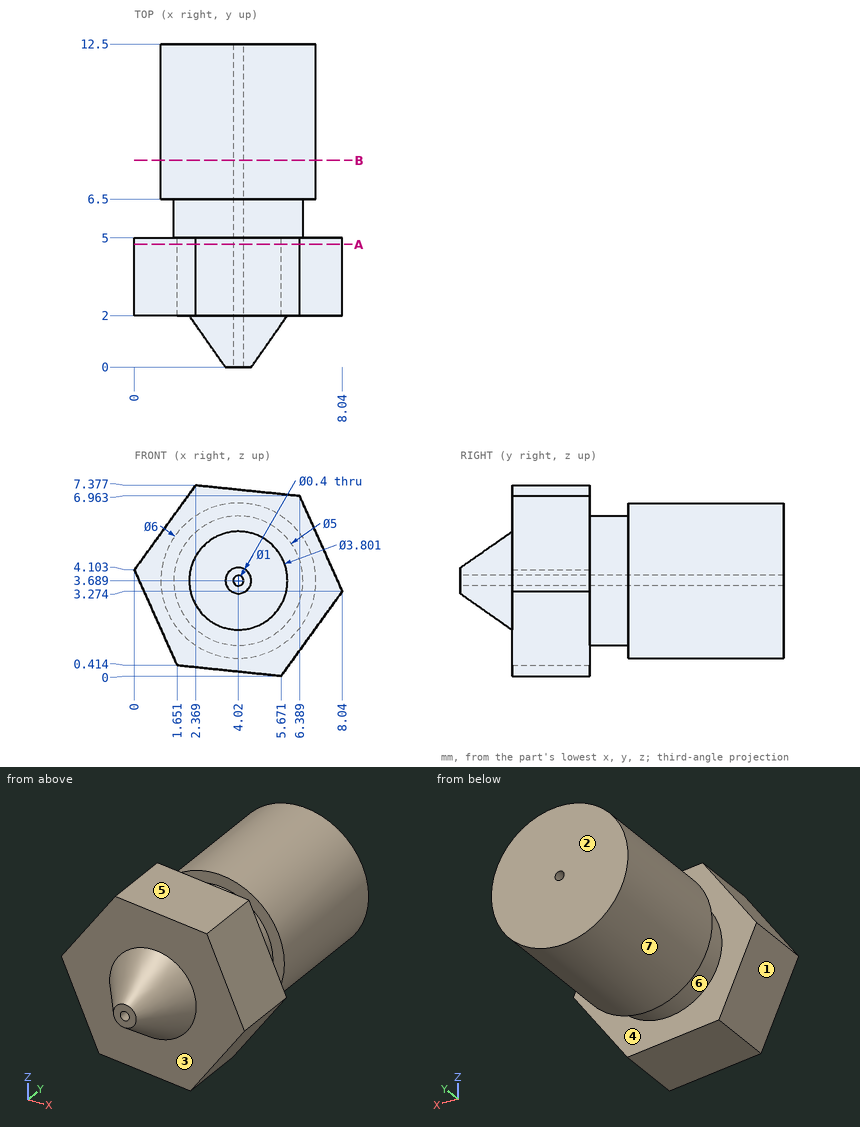
The drawing under review shows one solid part. Ordinate dimensions are in mm from its lowest x, y, z. A direction names the side the tool comes from. Round coordinates to 2 decimals unless told otherwise and drop trailing zeros. Order: outer loops, then holes, each group sorted by start corner. A loop starts at its lowest first (then second) coordinate and runs counter-clockwise, first axis right, second up. Notation, with made-up numbers: (-34.75, 36.5) -> (4.25, 36.5) arc R26 cw to (4.25, 67.5) -> close; hole circle Ø8 at (-14.75, 12.25). An arc over 180 degrees is marked (long way). Use a Markdown table: item, result.
Item 1: Draft analysis for pull direction Y (two halves, no side actions). For the marked faces 1, 2, 3 and 4, state which applies: +Y half, -Y half, draft (parallel to the pull), parting line (faces both ways), or undercut.
Resolved:
| item | result |
|---|---|
| face 1 | draft |
| face 2 | +Y half |
| face 3 | -Y half |
| face 4 | undercut |
Item 2: For pin 1 (1.5 mm diameter, centred on x = 2.5, z = 4, fed in from -Y); pin 2 (1 mm diameter, centred on y = 10, z = 5.5, fed in from -X); pin 3 (2 mm diameter, centred on x = 3.5, z = 2.5, fed in from -Y); pin 4 (2 mm diameter, centred on y = 9, z = 2.5, fed in from +X), all flat-tipped, find the tip position at first contact; note any pin that passes through.
Resolved:
| item | result |
|---|---|
| pin 1 | stops at y = 0.43 |
| pin 2 | stops at x = 1.32 |
| pin 3 | stops at y = 0 |
| pin 4 | stops at x = 7.01 |
Item 3: Take a section at B-B (y = 8). State the section outline as (x, z) points.
Resolved:
| item | result |
|---|---|
| outline | circle Ø6 at (4.02, 3.69); hole circle Ø0.4 at (4.02, 3.69) |
Item 4: For line 1 along Y through (x, z) = (3.75, 6.25); line 2 along Y through (x, z) = (5.75, 1); line 3 along Y through (x, z) = (3, 2), list the stretches that pass through material, from the lowest coordinate up. Write a range as [from, to].
Resolved:
| item | result |
|---|---|
| line 1 | y = [2, 5], [6.5, 12.5] |
| line 2 | y = [2, 5] |
| line 3 | y = [2, 12.5] |
Item 5: Machinability: for the marked faces 5, 6 and 7, which of the approach directions +Z, -Z, +X, -X, +Y, -Y give a long, thin tool a straight path to every point of the face, cutting with its end or side? Answer none if there is none.
Resolved:
| item | result |
|---|---|
| face 5 | +Z, +X, +Y, -Y |
| face 6 | none |
| face 7 | +Y |
Item 6: Take a section at A-A (y = 4.75). State the section outline as (x, z) points (1 decimal), plus the area to 3 significant figures.
Resolved:
| item | result |
|---|---|
| outline | (0, 4.1) -> (1.7, 0.4) -> (5.7, 0) -> (8, 3.3) -> (6.4, 7) -> (2.4, 7.4) -> close; hole circle Ø0.4 at (4, 3.7) |
| area | 42.3 mm² |
